Part model, mm, in its own coordinate system. Face numbers are marked on the shaded views. A direction names the side the tool comes from. Round coordinates to 2 decimals unless told otherwise and drop trailing zeros. Loops run counter-clockwise (first coordinate to the right, second up) from the corner with the lowest first, then second, coordinate; pieces in that order, holes last. Notation, with made-up numbers: (39, -35) - (96, -35) arc R22 ccw to (96, -22) - close; hole circle Ø2 at (-30.5, 72.25). An arc over 180 degrees is marked (long way). Write each question's results on one line, items separated by ' | '. Start each with the question number.
(1) Cut at D-D, the plane z = 15. List the corners of the cut face in (x, y), then the cut area to 3 significant figures.
(2) Cut at C-C, the plane x = -2.5. List the corners of the cut face in (y, z), then the cut area to 3 significant figures.
(3) Cut at A-A, the plane y = 0. List the corners of the cut face in (x, z).
(4) Cut at B-B, the plane x = 7.62. List the corners of the cut face in (y, z), then the cut area to 3 significant figures.
(5) Tool access for the marked faces 1, 2, 3 and 4: list every direction of +Z, -Z, +X, -X, +Y, -Y with a clear straight run to the whole face (end or side of a thin tool).
(6) Flat gauge pins, fed straight in: P1, Ø2.5, axis at x = 7.5, y = 2, coming from the +Z side; P2, Ø10, axis at y = -1, z = 29, coming from the -X side; P3, Ø6, axis at x = 1, y = -31.5, coming from the -Z side. Where does each tip first touch, or does it go through?
(7) Drill centre lines: L1, parallel to Y at x = 7.62, z = 2.25; L2, parallel to Z at x = -1.25, y = -35.5; L3, parallel to X at y = -50, z = 39. Where is each one in solid material? Low to high.
from build123d import *

# Parameters (mm, degrees)
SKETCH3_W           = 20.32
SKETCH3_H           = 12.7
BOSS_EXTRUDE1_DEPTH = 3.81
SKETCH4_R           = 1.778
CUT_EXTRUDE1_DEPTH  = 3.81
SKETCH5_W           = 7.62
SKETCH5_H           = 12.7
BOSS_EXTRUDE2_DEPTH = 25.4
FILLET1_R           = 1.27
FILLET2_R           = 1.27
BOSS_EXTRUDE6_DEPTH = 7.62
FILLET5_R           = 5.08
FILLET6_R           = 5.08
FILLET7_R           = 3.81


with BuildPart() as part:
    # Sketch3 → Boss-Extrude1 (new body)
    with BuildSketch(Plane.XY):
        Rectangle(SKETCH3_W, SKETCH3_H)
    extrude(amount=BOSS_EXTRUDE1_DEPTH)

    # Sketch4 → Cut-Extrude1 (cut)
    with BuildSketch(Plane.XY.offset(3.81)):
        with Locations((-7.62, 0)):
            Circle(SKETCH4_R)
        with Locations((7.62, 0)):
            Circle(SKETCH4_R)
    extrude(amount=-CUT_EXTRUDE1_DEPTH, mode=Mode.SUBTRACT)

    # Sketch5 → Boss-Extrude2 (add)
    with BuildSketch(Plane.XY.offset(3.81)):
        Rectangle(SKETCH5_W, SKETCH5_H)
    extrude(amount=BOSS_EXTRUDE2_DEPTH)

    # Fillet1
    fillet1_edges = [part.edges().sort_by_distance(p)[0] for p in [
        (-3.81, 0, 3.81),
    ]]
    fillet(fillet1_edges, radius=FILLET1_R)

    # Fillet2
    fillet2_edges = [part.edges().sort_by_distance(p)[0] for p in [
        (3.81, 0, 3.81),
    ]]
    fillet(fillet2_edges, radius=FILLET2_R)

    # Sketch10 → Boss-Extrude6 (add)
    with BuildSketch(Plane.ZY.offset(3.81)):
        Polygon((29.21, 6.35), (29.21, -57.15), (50.347792279, -58.999317196), (50.347792279, -56.459317196), (35.56, -44.45), (35.56, 6.35), align=None)
    extrude(amount=-BOSS_EXTRUDE6_DEPTH)

    # Fillet5
    fillet5_edges = [part.edges().sort_by_distance(p)[0] for p in [
        (0, -6.35, 29.21),
    ]]
    fillet(fillet5_edges, radius=FILLET5_R)

    # Fillet6
    fillet6_edges = [part.edges().sort_by_distance(p)[0] for p in [
        (0, 6.35, 35.56),
    ]]
    fillet(fillet6_edges, radius=FILLET6_R)

    # Fillet7
    fillet7_edges = [part.edges().sort_by_distance(p)[0] for p in [
        (0, -44.45, 35.56),
    ]]
    fillet(fillet7_edges, radius=FILLET7_R)


solid = part.part
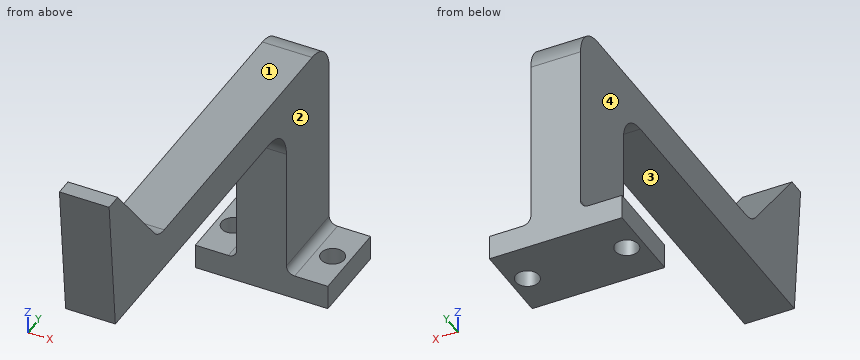
A:
1) outline: (-3.81, -6.35) - (3.81, -6.35) - (3.81, 6.35) - (-3.81, 6.35) - close | area: 96.8 mm2
2) outline: (-59, 50.35) - (-57.15, 29.21) - (-11.43, 29.21) arc R5.08 cw to (-6.35, 24.13) - (-6.35, 0) - (6.35, 0) - (6.35, 30.48) arc R5.08 ccw to (1.27, 35.56) - (-42.64, 35.56) arc R3.81 cw to (-45.59, 36.97) - (-56.46, 50.35) - close | area: 893 mm2
3) outline: (-10.16, 0) - (-9.4, 0) - (-9.4, 3.81) - (-10.16, 3.81) - close; (-5.84, 0) - (5.84, 0) - (5.84, 3.81) - (5.08, 3.81) arc R1.27 cw to (3.81, 5.08) - (3.81, 35.56) - (-3.81, 35.56) - (-3.81, 5.08) arc R1.27 cw to (-5.08, 3.81) - (-5.84, 3.81) - close; (9.4, 0) - (10.16, 0) - (10.16, 3.81) - (9.4, 3.81) - close
4) outline: (-6.35, 0) - (-1.78, 0) - (-1.78, 3.81) - (-6.35, 3.81) - close; (1.78, 0) - (6.35, 0) - (6.35, 3.81) - (1.78, 3.81) - close | area: 34.8 mm2
5) face 1: +Z, +X, -X, +Y | face 2: +Z, +X, +Y, -Y | face 3: -Z, +X, -X, -Y | face 4: +Z, -X, +Y, -Y
6) P1: z = 3.81 | P2: x = -3.81 | P3: z = 29.21
7) L1: -6.35 to -1.78, 1.78 to 6.35 | L2: 29.21 to 35.56 | L3: -3.81 to 3.81
